from build123d import *

# Parameters (mm, degrees)
SKETCH1_W                = 19.05
SKETCH1_H                = 22.225
BOSS_EXTRUDE1_DEPTH      = 3.175
SKETCH2_W                = 19.05
SKETCH2_H                = 3.175
BOSS_EXTRUDE2_DEPTH      = 21.59
F_1_4_CLEARANCE_HOLE2_D  = 6.7564
F_8_CLEARANCE_HOLE1_D    = 4.4958
MOVE_START               = -19.304
MOVE_FACE1_OUTLINE_W     = 19.05
MOVE_FACE1_OUTLINE_H     = 21.59
MOVE_FACE1_OUTLINE_R     = 2.2479
MOVE_FACE1_DEPTH         = 0.254
MOVE_START_2             = -22.225
MOVE_FACE1_2_OUTLINE_R   = 2.5019
MOVE_FACE1_2_OUTLINE_R_2 = 2.2479
MOVE_FACE1_2_DEPTH       = 2.921


# Read off the part's stored shape, not the designer's step: Move Face1
with BuildPart() as part:
    # Sketch1 → Boss-Extrude1 (new body)
    with BuildSketch(Plane(origin=(0, 0, 0), x_dir=(1, 0, 0), z_dir=(0, 1, 0))):
        with Locations((9.525, 11.1125)):
            Rectangle(SKETCH1_W, SKETCH1_H)
    extrude(amount=BOSS_EXTRUDE1_DEPTH)

    # Sketch2 → Boss-Extrude2 (add)
    with BuildSketch(Plane(origin=(0, 3.175, 0), x_dir=(1, 0, 0), z_dir=(0, 1, 0))):
        with Locations((9.525, 20.6375)):
            Rectangle(SKETCH2_W, SKETCH2_H)
    extrude(amount=BOSS_EXTRUDE2_DEPTH)

    # 1/4 Clearance Hole2 (through all)
    with Locations(Plane(origin=(9.525, 3.175, -6.35), x_dir=(0, 0, 1), z_dir=(0, 1, 0))):
        with Locations((0, 0)):
            Hole(F_1_4_CLEARANCE_HOLE2_D / 2)

    # #8 Clearance Hole1 (through all)
    with Locations(Plane(origin=(9.525, 15.24, -19.05), x_dir=(1, 0, 0), z_dir=(0, 0, 1))):
        with Locations((0, 0)):
            Hole(F_8_CLEARANCE_HOLE1_D / 2)

    # Move Face1 outline → Move Face1 (cut)
    with BuildSketch(Plane.XY.offset(MOVE_START)):
        with Locations((9.525, 13.97)):
            Rectangle(MOVE_FACE1_OUTLINE_W, MOVE_FACE1_OUTLINE_H)
        with Locations((9.525, 15.24)):
            Circle(MOVE_FACE1_OUTLINE_R, mode=Mode.SUBTRACT)
    extrude(amount=MOVE_FACE1_DEPTH, mode=Mode.SUBTRACT)

    # Move Face1 2 outline → Move Face1 2 (cut)
    with BuildSketch(Plane.XY.offset(MOVE_START_2)):
        with Locations((9.525, 15.24)):
            Circle(MOVE_FACE1_2_OUTLINE_R)
        with Locations((9.525, 15.24)):
            Circle(MOVE_FACE1_2_OUTLINE_R_2, mode=Mode.SUBTRACT)
    extrude(amount=MOVE_FACE1_2_DEPTH, mode=Mode.SUBTRACT)


solid = part.part
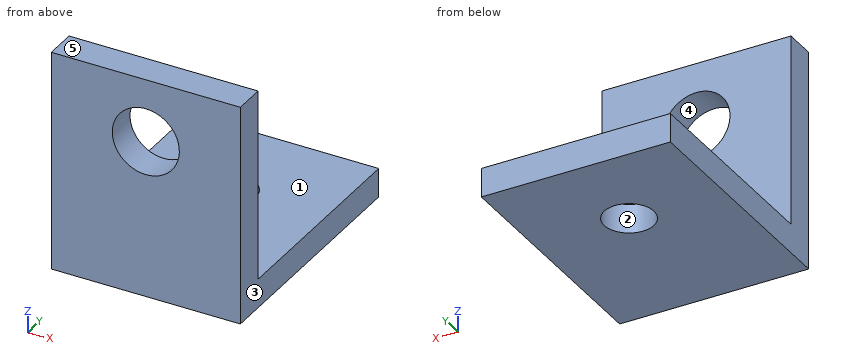
Input: part model. Units: mm. Frame: model coordinates. Face numbers are marked on the shaded views. A direction names the side the tool comes from. Coordinates: 2 decimals unless noted, no trailing zeros. Order: outer loops, then holes, each group sorted by start corner. A loop starts at its lowest first (then second) coordinate and runs counter-clockwise, first axis right, second up.
1. Draft query along X for the marked faces 3, 4 and 5. Return one class per face: +X half, -X half, draft (parallel to the pull), parting line (faces both ways), or undercut.
Checked values:
face 3: +X half
face 4: undercut
face 5: draft
2. Cut plane D-D, the plane y = 8. Return loops of the section in (x, z) (3 decimals).
Checked values:
outline: (0, -22.225) - (19.05, -22.225) - (19.05, -19.304) - (0, -19.304) - close
3. Cut plane A-A, the plane z = -6.35. Return loops of the section in (x, y) (3 decimals), plus the area to 3 significant figures.
Checked values:
outline: (0, 0) - (6.147, 0) - (6.147, 3.175) - (0, 3.175) - close; (12.903, 0) - (19.05, 0) - (19.05, 3.175) - (12.903, 3.175) - close
area: 39.0 mm2
4. Cut plane B-B, the plane y = 15.24. Return loops of the section in (x, z) (3 decimals).
Checked values:
outline: (0, -22.225) - (7.023, -22.225) - (7.023, -19.304) - (0, -19.304) - close; (12.027, -22.225) - (19.05, -22.225) - (19.05, -19.304) - (12.027, -19.304) - close
5. Ray query, line 1 along X through (y, z) = (2.25, -6.35); line 2 along Z through (x, y) = (11.75, 4.25) (3 decimals); line 3 along Y through (x, z) = (4, -9.75) (3 decimals). Return the intervals inside material, ascending.
Checked values:
line 1: x = 0 to 6.15, 12.9 to 19.05
line 2: z = -22.225 to -19.304
line 3: y = 0 to 3.175
6. Contact query for flat-ended pins moving along their axis: P1, Ø8, axis at x = 9.525, z = -6.35, coming from the +Y side (3 decimals); P2, Ø5, axis at x = 7.5, y = 14.5, coming from the +Z side. Output: stop coordinate, or through.
Checked values:
P1: stops at y = 3.175
P2: stops at z = -19.3
7. Cut plane C-C, the plane x = 3. Return loops of the section in (y, z) (3 decimals).
Checked values:
outline: (0, -22.225) - (24.765, -22.225) - (24.765, -19.304) - (3.175, -19.304) - (3.175, 0) - (0, 0) - close
8. Access query for the marked faces 1 and 2. Directions: +Z, -Z, +X, -X, +Y, -Y. A direction counts if a zero-diameter tool reaches every point of the face in a straight line with its end or side. Return the directions, or none.
Checked values:
face 1: +Z, +X, -X, +Y
face 2: +Z, -Z
